Part model, mm, in its own coordinate system. A direction names the side the tool comes from. Coordinates: 2 decimals unless noted, no trailing zeros. Order: outer loops, then holes, each group sorted by start corner. A loop starts at its lowest first (then second) coordinate and runs counter-clockwise, first axis right, second up.
1) Cut at A-A (x = 108). List the corners of the cut face in (y, z), and give its area (3 significant figures).
2) Cut at C-C (z = 46). List the corners of the cut face in (x, y), and give its area (3 significant figures).
3) Tool access for faces 1 (the flat face through (101, -16.51, 19)), 2 (the cylindrical face through (3.62, -9.66, 3.82)), 3 (the cylindrical face through (22.14, -17.76, 21.85)): list every direction of +Z, -Z, +X, -X, +Y, -Y with a clear straight run to the whole face (end or side of a thin tool).
4) Pin check, flat tips, straight feed: pin 1 Ø7 at (x, y) = (158.5, -9.5) entering from +Z; pin 2 Ø10 at (x, z) = (102, 80.5) entering from -Y; pin 3 Ø2 at (x, y) = (103, -17.5) entering from +Z. Stop position of each tip, or through.
5) Mould opens along Y. For faces 4 (the flat face through (100, 0, 59)), 5 (the flat face through (203.2, -9, 58)), 6 (the flat face through (190.5, -10, 67)) say: +Y half, -Y half, draft (parallel to the pull), parting line (faces both ways), or undercut.
6) Wall check: L1, parallel to X at y = -4.75, z = 38; L2, parallel to X at y = -16, z = 13; L3, parallel to Y at x = 119.5, z = 111. Give the ranges that are in metal, low to high.
7) Cut at D-D (x = 170). List the corners of the cut face in (y, z), and give its area (3 significant figures).
```python
from build123d import *

# Parameters (mm, degrees)
F0_W     = 203.2
F0_H     = 116.84
F1_DEPTH = 19.05
F2_W     = 177.8
F2_H     = 13.97
F3_DEPTH = 101.6
F4_W     = 161.8175851255
F4_H     = 96.52
F5_DEPTH = 2.54
F6_W     = 63.5
F6_H     = 13.97
F7_DEPTH = 15.241
F8_W     = 63.5
F8_H     = 12.7
F9_DEPTH = 19.051
F10_R    = 12.69999
F11_R    = 5.08


# Not quite as in the source:
# - a fillet or chamfer is up to 0.001 mm smaller than in the source, because OpenCascade refuses the exact size


with BuildPart() as f1:
    # F0 (on Front) → F1 (new body)
    with BuildSketch(Plane.XZ):
        with Locations((101.6, 58.42)):
            Rectangle(F0_W, F0_H)
    extrude(amount=F1_DEPTH)

    # F2 (on face) → F3 (cut)
    with BuildSketch(Plane.XY.offset(116.84)):
        with Locations((101.6, -9.525)):
            Rectangle(F2_W, F2_H)
    extrude(amount=-F3_DEPTH, mode=Mode.SUBTRACT)

    # F4 (on face) → F5 (cut, through all)
    with BuildSketch(Plane.XZ.offset(19.05)):
        with Locations((101.6, 68.58)):
            Rectangle(F4_W, F4_H)
    extrude(amount=-F5_DEPTH, mode=Mode.SUBTRACT)

    # F6 (on face) → F7 (cut, through all)
    with BuildSketch(Plane.XY.offset(15.24)):
        with Locations((101.6, -9.525)):
            Rectangle(F6_W, F6_H)
    extrude(amount=-F7_DEPTH, mode=Mode.SUBTRACT)

    # F8 (on face) → F9 (cut, through all)
    with BuildSketch(Plane.XZ.offset(19.05)):
        with Locations((101.6, 6.35)):
            Rectangle(F8_W, F8_H)
    extrude(amount=-F9_DEPTH, mode=Mode.SUBTRACT)

    # F10 (radius 12.7 in the source; OpenCascade refuses exactly that, so slightly less here)
    f10_edges = [f1.edges().sort_by_distance(p)[0] for p in [
        (0, -9.525, 116.84),
        (0, -9.525, 0),
        (203.2, -9.525, 0),
        (203.2, -9.525, 116.84),
    ]]
    fillet(f10_edges, radius=F10_R)

    # F11
    f11_edges = [f1.edges().sort_by_distance(p)[0] for p in [
        (20.691207, -17.78, 20.32),
        (182.508793, -17.78, 20.32),
    ]]
    fillet(f11_edges, radius=F11_R)


solid = f1.part
```
Geometry check:
1. outline: (-19.05, 12.7) - (-16.51, 12.7) - (-16.51, 20.32) - (-19.05, 20.32) - close; (-2.54, 12.7) - (0, 12.7) - (0, 116.84) - (-2.54, 116.84) - close
1. area: 284 mm2
2. outline: (0, -19.05) - (20.69, -19.05) - (20.69, -16.51) - (12.7, -16.51) - (12.7, -2.54) - (190.5, -2.54) - (190.5, -16.51) - (182.51, -16.51) - (182.51, -19.05) - (203.2, -19.05) - (203.2, 0) - (0, 0) - close
2. area: 976 mm2
3. face 1: +Z
3. face 2: -Z, -X, +Y, -Y
3. face 3: +Z, -Y
4. pin 1: stops at z = 15.24
4. pin 2: stops at y = -2.54
4. pin 3: stops at z = 20.32
5. face 4: +Y half
5. face 5: draft
5. face 6: undercut
6. L1: x = 0 to 12.7, 190.5 to 203.2
6. L2: x = 0 to 69.85, 133.35 to 203.2
6. L3: y = -2.54 to 0
7. outline: (-19.05, 0) - (0, 0) - (0, 116.84) - (-2.54, 116.84) - (-2.54, 15.24) - (-16.51, 15.24) - (-16.51, 20.32) - (-19.05, 20.32) - close
7. area: 561 mm2
